Source: CAD feature listing. Evaluate the final solid. Frame: model axes, mm. A direction names the side the tool comes from. Give positions to 0.01 mm unless a question says otherwise; leave off trailing zeros. Order: outer loops, then holes, each group sorted by start corner. A loop starts at its lowest first (then second) coordinate and runs counter-clockwise, first axis right, second up.
Autodesk Inventor part; units mm, degrees
ref_plane "YZ Plane" through (0, 0, 0) normal (1, 0, 0) x (0, 1, 0)
ref_plane "XZ Plane" through (0, 0, 0) normal (0, 1, 0) x (-1, 0, 0)
ref_plane "XY Plane" through (0, 0, 0) normal (0, 0, 1) x (1, 0, 0)
sketch "Sketch1" plane through (0, 0, 0) normal (0, 0, 1) x (1, 0, 0)
  line L0 (0, -40) -> (0, 0)
  line L1 (0, 0) -> (-130, 0)
  line L2 (-130, 0) -> (-330.7518, -286.7032)
  line L3 (-330.7518, -286.7032) -> (-330.7518, -735.1242)
  line L4 (-326.7518, -735.1242) -> (-326.7518, -287.9644)
  line L5 (-326.7518, -287.9644) -> (-127.9177, -4)
  line L6 (-127.9177, -4) -> (-4, -4)
  line L7 (-4, -4) -> (-4, -40)
  line L8 (-4, -40) -> (0, -40)
  line L9 (-330.7518, -735.1242) -> (-326.7518, -735.1242)
  dimension "d0" = 40
  dimension "d1" = 130
  dimension "d2" = 125
  dimension "d3" = 350
  dimension "d4" = 448.421
  dimension "d5" = 4
extrude "Extrusion1" add sketch "Sketch1" along normal blind 1200
properties part number "polycarbonate cover" material "Polycarbonate, Smoke"
1) First-contact query: pin 1 Ø5 at (x, z) = (-295, 1025.5) entering from +Y; pin 2 Ø6 at (x, z) = (-128.5, 1069) entering from -Y; pin 3 Ø8 at (x, z) = (-82, 206.5) entering from -Y. Flat tips, straight axial feed; report the tip coordinate or a pass-through.
Checks:
pin 1: stops at y = -232.07
pin 2: stops at y = -9.12
pin 3: stops at y = -4
2) Section query A-A on z = 695. Output: boundary loops of the cut face in (x, y), and give its area (3 significant figures).
Checks:
outline: (-330.75, -735.12) - (-326.75, -735.12) - (-326.75, -287.96) - (-127.92, -4) - (-4, -4) - (-4, -40) - (0, -40) - (0, 0) - (-130, 0) - (-330.75, -286.7) - close
area: 3,840 mm2
3) Section query C-C on x = -257. Output: boundary loops of the cut face in (y, z).
Checks:
outline: (-188.35, 0) - (-181.37, 0) - (-181.37, 1200) - (-188.35, 1200) - close
4) Pull-direction query (X, two-part tool) for faces 1 (the face through (0, -20, 592)), 2 (the face through (-67, -4, 592)), 3 (the face through (-228.971, -141.345, 591.6)); classes: +X half, -X half, draft (parallel to the pull), parting line (faces both ways), or undercut.
Checks:
face 1: +X half
face 2: undercut
face 3: -X half
5) Ray query, L1, parallel to X at y = -472, z = 1003; L2, parallel to Y at x = -107.5, z = 1120; L3, parallel to Y at x = -155, z = 1058. Return the intervals inside material, ascending.
Checks:
L1: x = -330.75 to -326.75
L2: y = -4 to 0
L3: y = -42.68 to -35.7
6) Section query B-B on y = -479.5. Output: boundary loops of the cut face in (x, z), and give its area (3 significant figures).
Checks:
outline: (-330.75, 0) - (-326.75, 0) - (-326.75, 1200) - (-330.75, 1200) - close
area: 4,800 mm2
7) Reachability of faces 4 (the face through (-64, 0, 592)), 5 (the face through (-4, -22, 592)), 6 (the face through (-326.752, -515, 592)) from +Z, -Z, +X, -X, +Y, -Y: full face, straight path, thin tool, end or side. Return the list, or none.
Checks:
face 4: +Z, -Z, +X, -X, +Y
face 5: +Z, -Z, -Y
face 6: +Z, -Z, +X, -Y
